Verification items for the finished model (mm, model axes). Give positions to 0.01 mm unless a question says otherwise; leave off trailing zeros. Order: outer loops, then holes, each group sorted by start corner. A loop starts at its lowest first (then second) coordinate and runs counter-clockwise, first axis right, second up.
(1) Sectioned sample at A-A on x = -109.6. Record the cut outline in (y, z).
(2) Scan lines: L1, parallel to Z at x = -152, y = -4; L2, parallel to Z at x = -34.8, y = -4.5; L3, parallel to X at y = -2.75, z = 7.5. Record each from-to range of solid material in increasing order.
(3) Mould release check, pull along X, two halves, no side actions. Record for faces 1 (the face through (191, -5, -25)), 2 (the face through (-30.985, -4.93, 1.201)): pulls with the +X half, pulls with the -X half, needs draft (parallel to the pull), parting line crosses it, or undercut.
(4) Gauge pin test, flat ends, axial feed: pin 1 (5.5 mm diameter, centred on x = 62.5, z = 0, fed in from -Y); pin 2 (3 mm diameter, centred on x = 110, y = -4.5, fed in from -Z); pin 3 (3 mm diameter, centred on y = -3.5, z = -22.5, fed in from -X); pin 4 (4.5 mm diameter, centred on y = -3, z = 23, fed in from +X). Record the tip position at first contact, or that the pin passes through.
```python
from build123d import *

# Parameters (mm, degrees)
F0_R         = 10
F0_R_2       = 3
F0_R_3       = 5
F0_R_4       = 4
F1_DEPTH     = 10
F2_T1_DEPTH  = 22
F2_T3_DEPTH  = 23.6
F2_T5_DEPTH  = 11.5
F2_T7_DEPTH  = 373.8
F2_T9_DEPTH  = 11.5
F2_T11_DEPTH = 23.6
F2_T14_ANGLE = 71.0490813257
F2_T16_ANGLE = 71.0490813257
F2_T18_ANGLE = 71.0490813257
F2_T20_ANGLE = 71.0490813257
F2_T25_DEPTH = 19
F2_T29_DEPTH = 381.3
F2_T36_DEPTH = 381.3
F2_T40_DEPTH = 19
F2_T47_DEPTH = 19
F2_T51_DEPTH = 381.3
F2_T58_DEPTH = 381.3
F2_T62_DEPTH = 19


# Not quite as in the source:
# - a fillet or chamfer that OpenCascade refuses, or shapes differently, is made with other operations: its cross-section is extruded or revolved along the edge and cut away or added


with BuildPart() as f1:
    # F0 (on Front) → F1 (new body)
    with BuildSketch(Plane.XZ):
        with BuildLine():
            ThreePointArc((251, 3.5), (220.5089399385, 7.1742403064), (195.5, 25))
            Line((195.5, 25), (186.9, 25))
            Line((186.9, 25), (186.9, 21))
            Line((186.9, 21), (-186.9, 21))
            Line((-186.9, 21), (-186.9, 25))
            Line((-186.9, 25), (-195.5, 25))
            ThreePointArc((-195.5, 25), (-220.5089399385, 7.1742403064), (-251, 3.5))
            Line((-251, 3.5), (-251, -3.5))
            ThreePointArc((-251, -3.5), (-220.5089399385, -7.1742403064), (-195.5, -25))
            Line((-195.5, -25), (-186.9, -25))
            Line((-186.9, -25), (-186.9, -21))
            Line((-186.9, -21), (186.9, -21))
            Line((186.9, -21), (186.9, -25))
            Line((186.9, -25), (195.5, -25))
            ThreePointArc((195.5, -25), (220.5089399385, -7.1742403064), (251, -3.5))
            Line((251, -3.5), (251, 3.5))
        make_face()
        with Locations((-201, 0)):
            Circle(F0_R, mode=Mode.SUBTRACT)
        with Locations((-152, 0)):
            Circle(F0_R_2, mode=Mode.SUBTRACT)
        with Locations((-109.6, 0)):
            Circle(F0_R_3, mode=Mode.SUBTRACT)
        with Locations((-71, 0)):
            Circle(F0_R_2, mode=Mode.SUBTRACT)
        with Locations((-34.8, 0)):
            Circle(F0_R_4, mode=Mode.SUBTRACT)
        with Locations((16.5, 0)):
            Circle(F0_R_2, mode=Mode.SUBTRACT)
        with Locations((62.5, 0)):
            Circle(F0_R_2, mode=Mode.SUBTRACT)
        with Locations((103.2, 0)):
            Circle(F0_R_2, mode=Mode.SUBTRACT)
        with Locations((142.5, 0)):
            Circle(F0_R_3, mode=Mode.SUBTRACT)
        with Locations((194.1, 0)):
            Circle(F0_R, mode=Mode.SUBTRACT)
    extrude(amount=F1_DEPTH)

    # F2: fillet of radius 3 on 15 edges, made by hand

    # F2_s2 → F2_t1 (cut)
    with BuildSketch(Plane.XY.offset(-11)):
        with BuildLine():
            ThreePointArc((251, -7), (250.1213203436, -9.1213203436), (248, -10))
            Line((248, -10), (251, -10))
            Line((251, -10), (251, -7))
        make_face()
        with BuildLine():
            ThreePointArc((-251, -7), (-250.1213203436, -9.1213203436), (-248, -10))
            Line((-248, -10), (-251, -10))
            Line((-251, -10), (-251, -7))
        make_face()
    extrude(amount=F2_T1_DEPTH, mode=Mode.SUBTRACT)

    # F2_s4 → F2_t3 (cut)
    with BuildSketch(Plane.YZ.offset(179.4)):
        with BuildLine():
            ThreePointArc((-7, 25), (-9.1213203436, 24.1213203436), (-10, 22))
            Line((-10, 22), (-10, 25))
            Line((-10, 25), (-7, 25))
        make_face()
    extrude(amount=F2_T3_DEPTH, mode=Mode.SUBTRACT)

    # F2_s6 → F2_t5 (cut)
    with BuildSketch(Plane.XY.offset(21)):
        with BuildLine():
            ThreePointArc((186.9, -7), (187.7786796564, -9.1213203436), (189.9, -10))
            Line((189.9, -10), (186.9, -10))
            Line((186.9, -10), (186.9, -7))
        make_face()
        with BuildLine():
            ThreePointArc((-186.9, -7), (-187.7786796564, -9.1213203436), (-189.9, -10))
            Line((-189.9, -10), (-186.9, -10))
            Line((-186.9, -10), (-186.9, -7))
        make_face()
    extrude(amount=F2_T5_DEPTH, mode=Mode.SUBTRACT)

    # F2_s8 → F2_t7 (cut)
    with BuildSketch(Plane.YZ.offset(-186.9)):
        with BuildLine():
            ThreePointArc((-7, 21), (-9.1213203436, 20.1213203436), (-10, 18))
            Line((-10, 18), (-10, 21))
            Line((-10, 21), (-7, 21))
        make_face()
        with BuildLine():
            ThreePointArc((-7, -21), (-9.1213203436, -20.1213203436), (-10, -18))
            Line((-10, -18), (-10, -21))
            Line((-10, -21), (-7, -21))
        make_face()
    extrude(amount=F2_T7_DEPTH, mode=Mode.SUBTRACT)

    # F2_s10 → F2_t9 (cut)
    with BuildSketch(Plane.XY.offset(-32.5)):
        with BuildLine():
            ThreePointArc((186.9, -7), (187.7786796564, -9.1213203436), (189.9, -10))
            Line((189.9, -10), (186.9, -10))
            Line((186.9, -10), (186.9, -7))
        make_face()
        with BuildLine():
            ThreePointArc((-186.9, -7), (-187.7786796564, -9.1213203436), (-189.9, -10))
            Line((-189.9, -10), (-186.9, -10))
            Line((-186.9, -10), (-186.9, -7))
        make_face()
    extrude(amount=F2_T9_DEPTH, mode=Mode.SUBTRACT)

    # F2_s12 → F2_t11 (cut)
    with BuildSketch(Plane.YZ.offset(-203)):
        with BuildLine():
            ThreePointArc((-7, 25), (-9.1213203436, 24.1213203436), (-10, 22))
            Line((-10, 22), (-10, 25))
            Line((-10, 25), (-7, 25))
        make_face()
        with BuildLine():
            ThreePointArc((-7, -25), (-9.1213203436, -24.1213203436), (-10, -22))
            Line((-10, -22), (-10, -25))
            Line((-10, -25), (-7, -25))
        make_face()
    extrude(amount=F2_T11_DEPTH, mode=Mode.SUBTRACT)

    # F2_s13 → F2_t14 (revolve, cut)
    with BuildSketch(Plane(origin=(243.6742780769, 0, 62.3328752784), x_dir=(0, 1, 0), z_dir=(0.9688050004, 0, 0.2478242748))):
        with BuildLine():
            ThreePointArc((-7, -59.2652075087), (-9.1213203436, -60.1438871651), (-10, -62.2652075087))
            Line((-10, -62.2652075087), (-10, -59.2652075087))
            Line((-10, -59.2652075087), (-7, -59.2652075087))
        make_face()
    revolve(axis=Axis((242.9593619468, -10, 65.127655258), (0, 1, 0)), revolution_arc=F2_T14_ANGLE, mode=Mode.SUBTRACT)

    # F2_s15 → F2_t16 (revolve, cut)
    with BuildSketch(Plane(origin=(43.3477149421, 0, 65.9912921941), x_dir=(0, 1, 0), z_dir=(-0.5490187323, 0, -0.8358100452))):
        with BuildLine():
            ThreePointArc((-7, 176.6742001078), (-9.1213203436, 175.7955204514), (-10, 173.6742001078))
            Line((-10, 173.6742001078), (-10, 176.6742001078))
            Line((-10, 176.6742001078), (-7, 176.6742001078))
        make_face()
    revolve(axis=Axis((242.9593619468, -10, -65.127655258), (0, 1, 0)), revolution_arc=F2_T16_ANGLE, mode=Mode.SUBTRACT)

    # F2_s17 → F2_t18 (revolve, cut)
    with BuildSketch(Plane(origin=(-243.6742780769, 0, -62.3328752784), x_dir=(0, 1, 0), z_dir=(-0.9688050004, 0, -0.2478242748))):
        with BuildLine():
            ThreePointArc((-7, -59.2652075087), (-9.1213203436, -60.1438871651), (-10, -62.2652075087))
            Line((-10, -62.2652075087), (-10, -59.2652075087))
            Line((-10, -59.2652075087), (-7, -59.2652075087))
        make_face()
    revolve(axis=Axis((-242.9593619468, -10, -65.127655258), (0, 1, 0)), revolution_arc=F2_T18_ANGLE, mode=Mode.SUBTRACT)

    # F2_s19 → F2_t20 (revolve, cut)
    with BuildSketch(Plane(origin=(-43.3477149421, 0, -65.9912921941), x_dir=(0, 1, 0), z_dir=(0.5490187323, 0, 0.8358100452))):
        with BuildLine():
            ThreePointArc((-7, 176.6742001078), (-9.1213203436, 175.7955204514), (-10, 173.6742001078))
            Line((-10, 173.6742001078), (-10, 176.6742001078))
            Line((-10, 176.6742001078), (-7, 176.6742001078))
        make_face()
    revolve(axis=Axis((-242.9593619468, -10, 65.127655258), (0, 1, 0)), revolution_arc=F2_T20_ANGLE, mode=Mode.SUBTRACT)


with BuildPart() as f2_tool23:
    # F2_s24 → F2_t25 (new body)
    with BuildSketch(Plane.XY.offset(32.5)):
        with BuildLine():
            ThreePointArc((186.9, -7), (187.7786796564, -9.1213203436), (189.9, -10))
            Line((189.9, -10), (186.9, -10))
            Line((186.9, -10), (186.9, -7))
        make_face()
    extrude(amount=-F2_T25_DEPTH)

    split(bisect_by=Plane.XY.offset(21), keep=Keep.BOTTOM)


with BuildPart() as f2_tool27:
    # F2_s28 → F2_t29 (new body)
    with BuildSketch(Plane.YZ.offset(194.4)):
        with BuildLine():
            ThreePointArc((-7, 21), (-9.1213203436, 20.1213203436), (-10, 18))
            Line((-10, 18), (-10, 21))
            Line((-10, 21), (-7, 21))
        make_face()
    extrude(amount=-F2_T29_DEPTH)

    split(bisect_by=Plane.YZ.offset(186.9), keep=Keep.TOP)


with BuildPart() as f2_tool23_1:
    add(f2_tool23.part)

    # F2_t31: intersect F2_tool27
    add(f2_tool27.part, mode=Mode.INTERSECT)


with BuildPart() as f1_1:
    add(f1.part)

    # F2_t21: cut F2_tool23
    add(f2_tool23_1.part, mode=Mode.SUBTRACT)


with BuildPart() as f2_tool34:
    # F2_s35 → F2_t36 (new body)
    with BuildSketch(Plane.YZ.offset(186.9)):
        with BuildLine():
            ThreePointArc((-7, 21), (-9.1213203436, 20.1213203436), (-10, 18))
            Line((-10, 18), (-10, 21))
            Line((-10, 21), (-7, 21))
        make_face()
    extrude(amount=-F2_T36_DEPTH)

    split(bisect_by=Plane.YZ.offset(-186.9), keep=Keep.BOTTOM)


with BuildPart() as f2_tool38:
    # F2_s39 → F2_t40 (new body)
    with BuildSketch(Plane.XY.offset(13.5)):
        with BuildLine():
            ThreePointArc((-186.9, -7), (-187.7786796564, -9.1213203436), (-189.9, -10))
            Line((-189.9, -10), (-186.9, -10))
            Line((-186.9, -10), (-186.9, -7))
        make_face()
    extrude(amount=F2_T40_DEPTH)

    split(bisect_by=Plane.XY.offset(21), keep=Keep.BOTTOM)


with BuildPart() as f2_tool34_1:
    add(f2_tool34.part)

    # F2_t42: intersect F2_tool38
    add(f2_tool38.part, mode=Mode.INTERSECT)


with BuildPart() as f1_2:
    add(f1_1.part)

    # F2_t32: cut F2_tool34
    add(f2_tool34_1.part, mode=Mode.SUBTRACT)


with BuildPart() as f2_tool45:
    # F2_s46 → F2_t47 (new body)
    with BuildSketch(Plane.XY.offset(-32.5)):
        with BuildLine():
            ThreePointArc((-186.9, -7), (-187.7786796564, -9.1213203436), (-189.9, -10))
            Line((-189.9, -10), (-186.9, -10))
            Line((-186.9, -10), (-186.9, -7))
        make_face()
    extrude(amount=F2_T47_DEPTH)

    split(bisect_by=Plane.XY.offset(-21), keep=Keep.TOP)


with BuildPart() as f2_tool49:
    # F2_s50 → F2_t51 (new body)
    with BuildSketch(Plane.YZ.offset(-194.4)):
        with BuildLine():
            ThreePointArc((-7, -21), (-9.1213203436, -20.1213203436), (-10, -18))
            Line((-10, -18), (-10, -21))
            Line((-10, -21), (-7, -21))
        make_face()
    extrude(amount=F2_T51_DEPTH)

    split(bisect_by=Plane.YZ.offset(-186.9), keep=Keep.BOTTOM)


with BuildPart() as f2_tool45_1:
    add(f2_tool45.part)

    # F2_t53: intersect F2_tool49
    add(f2_tool49.part, mode=Mode.INTERSECT)


with BuildPart() as f1_3:
    add(f1_2.part)

    # F2_t43: cut F2_tool45
    add(f2_tool45_1.part, mode=Mode.SUBTRACT)


with BuildPart() as f2_tool56:
    # F2_s57 → F2_t58 (new body)
    with BuildSketch(Plane.YZ.offset(-186.9)):
        with BuildLine():
            ThreePointArc((-7, -21), (-9.1213203436, -20.1213203436), (-10, -18))
            Line((-10, -18), (-10, -21))
            Line((-10, -21), (-7, -21))
        make_face()
    extrude(amount=F2_T58_DEPTH)

    split(bisect_by=Plane.YZ.offset(186.9), keep=Keep.TOP)


with BuildPart() as f2_tool60:
    # F2_s61 → F2_t62 (new body)
    with BuildSketch(Plane.XY.offset(-13.5)):
        with BuildLine():
            ThreePointArc((186.9, -7), (187.7786796564, -9.1213203436), (189.9, -10))
            Line((189.9, -10), (186.9, -10))
            Line((186.9, -10), (186.9, -7))
        make_face()
    extrude(amount=-F2_T62_DEPTH)

    split(bisect_by=Plane.XY.offset(-21), keep=Keep.TOP)


with BuildPart() as f2_tool56_1:
    add(f2_tool56.part)

    # F2_t64: intersect F2_tool60
    add(f2_tool60.part, mode=Mode.INTERSECT)


with BuildPart() as f1_4:
    add(f1_3.part)

    # F2_t54: cut F2_tool56
    add(f2_tool56_1.part, mode=Mode.SUBTRACT)


solid = f1_4.part
```
Ans:
1. outline: (-10, -18) arc R3 ccw to (-7, -21) - (0, -21) - (0, -5) - (-10, -5) - close; (-10, 5) - (0, 5) - (0, 21) - (-7, 21) arc R3 ccw to (-10, 18) - close
2. L1: z = -21 to -3, 3 to 21
2. L2: z = -21 to -4, 4 to 21
2. L3: x = -219.69 to -207.61, -194.39 to 187.49, 200.71 to 219.69
3. face 1: needs draft
3. face 2: undercut
4. pin 1: passes through
4. pin 2: stops at z = -21
4. pin 3: stops at x = -199.19
4. pin 4: stops at x = 199.45
